Build history of the part. All positions in model axes, mm. Give positions to 0.01 mm unless a question says otherwise; leave off trailing zeros. Write each loop counter-clockwise with the first axis right and the second up, starting at its lowest first coordinate (ties: lowest second). Pieces come first, ordered by that corner, then holes. Notation, with made-up numbers: (68.5, 70) -> (126.5, 70) arc R9 cw to (126.5, 78) -> close; hole circle Ø7 at (77.5, -23.5). An arc over 180 degrees is marked (long way). One line per question, with ' | ' between items. Start each with the question number.
(1) Pin check, flat tips, straight feed: P1, Ø1.5, axis at y = -239, z = 1.5, coming from the -X side; P2, Ø3.5, axis at x = -7.21, y = -91.25, coming from the -Z side. Stop position of each tip, or through.
(2) Band-saw the part on A-A, the plane y = -238.75. Give the cut face in (x, z).
(3) Band-saw the part on B-B, the plane z = 0.6. Count the separate pieces of the cut face and the enclosed holes in it, and give its area (3 significant figures).
(4) Pull direction Y, two halves, no side cores. Call faces 1 (the flat face through (-8, -164, 3)), 2 (the cylindrical face through (67.467, -199.274, 1.479)): released by +Y, released by -Y, zero draft, split by the parting line, or undercut.
(5) Drill centre lines: probe 1 along X at (y, z) = (-197.5, 1.5); probe 2 along Y at (x, z) = (65.5, 1.2); probe 3 along X at (y, z) = (-238.75, 1.2). Where is each one in solid material? Low to high. Write a range as from..to.
(6) Band-saw the part on C-C, the plane y = -197.5. Give the cut face in (x, z).
(7) Band-saw the part on D-D, the plane y = -91.25. Give the cut face in (x, z).
from build123d import *

# Parameters (mm, degrees)
ESQUISSE1_R        = 2
BOSS_EXTRU_1_DEPTH = 3


with BuildPart() as part:
    # Esquisse1 → Boss.-Extru.1 (new body)
    with BuildSketch(Plane.XY):
        Polygon((-89.706165703, -247.5), (75.293834297, -247.5), (75.293834297, -242.5), (65.293834297, -242.5), (65.293834297, -232.5), (75.293834297, -232.5), (75.293834297, -162.5), (65.293834297, -162.5), (65.293834297, -152.5), (75.293834297, -152.5), (75.293834297, -131.583123952), (65.293834297, -131.583123952), (65.293834297, -98.416876048), (75.293834297, -98.416876048), (75.293834297, -82.5), (-89.706165703, -82.5), (-89.706165703, -98.416876048), (-79.706165703, -98.416876048), (-79.706165703, -131.583123952), (-89.706165703, -131.583123952), (-89.706165703, -152.5), (-79.706165703, -152.5), (-79.706165703, -162.5), (-89.706165703, -162.5), (-89.706165703, -232.5), (-79.706165703, -232.5), (-79.706165703, -242.5), (-89.706165703, -242.5), align=None)
        with Locations((-7.206165703, -91.25)):
            Circle(ESQUISSE1_R, mode=Mode.SUBTRACT)
        with Locations((-80.956165703, -197.5)):
            Circle(ESQUISSE1_R, mode=Mode.SUBTRACT)
        with Locations((-7.206165703, -238.75)):
            Circle(ESQUISSE1_R, mode=Mode.SUBTRACT)
        with Locations((66.543834297, -197.5)):
            Circle(ESQUISSE1_R, mode=Mode.SUBTRACT)
    extrude(amount=BOSS_EXTRU_1_DEPTH)


solid = part.part
Results:
1) P1: stops at x = -79.71 | P2: passes through
2) outline: (-79.71, 0) -> (-9.21, 0) -> (-9.21, 3) -> (-79.71, 3) -> close; (-5.21, 0) -> (65.29, 0) -> (65.29, 3) -> (-5.21, 3) -> close
3) separate pieces: 1 | enclosed holes: 4 | area: 26,100 mm²
4) face 1: zero draft | face 2: undercut
5) probe 1: x = -89.71..-82.96, -78.96..64.54, 68.54..75.29 | probe 2: y = -247.5..-242.5, -232.5..-199.21, -195.79..-162.5, -152.5..-131.58, -98.42..-82.5 | probe 3: x = -79.71..-9.21, -5.21..65.29
6) outline: (-89.71, 0) -> (-82.96, 0) -> (-82.96, 3) -> (-89.71, 3) -> close; (-78.96, 0) -> (64.54, 0) -> (64.54, 3) -> (-78.96, 3) -> close; (68.54, 0) -> (75.29, 0) -> (75.29, 3) -> (68.54, 3) -> close
7) outline: (-89.71, 0) -> (-9.21, 0) -> (-9.21, 3) -> (-89.71, 3) -> close; (-5.21, 0) -> (75.29, 0) -> (75.29, 3) -> (-5.21, 3) -> close
